Can you work these out from the model? Positions are in its coordinate system, mm. Face numbers are marked on the shaded views. A direction names the side the tool comes from. Coordinates: 2 decimals unless noted, no trailing zeros. Order: outer loops, then holes, each group sorted by start corner. A loop starts at its lowest first (then second) coordinate and runs counter-clockwise, first axis right, second up. Notation, with made-up numbers: (83, 47.5) -> (114, 47.5) arc R20 ccw to (114, 58.5) -> close; hole circle Ø4 at (-30.5, 64). An arc over 180 degrees is marked (long way). Return JSON: item names as keys, results as strings. Group by question number.
1) If I drill on probe 1 along X at (y, z) = (5, 1.6); probe 2 along Y at (x, z) = (17, 3); probe 3 along Y at (x, z) = (89, 1.1), over which ranges is the centre line in solid material (lowest first)? Write a range as from..to.
2) If we section it at A-A, the plane x = 17: Please give me the cut outline in (y, z).
3) For the marked faces 1, 2, 3 and 4, which set-ups out of +Z, -Z, +X, -X, +Y, -Y let a thin tool reach every point of the face, with its end or its side?
4) If we section it at B-B, the plane z = 3: State how many separate pieces and enclosed holes the cut face has, then the cut area to 3 significant figures.
5) For pin 1 (1.8 mm diameter, centred on x = 64, y = 58.5, fed in from +Z); pin 2 (5.5 mm diameter, centred on x = 65, y = 5, fed in from -Z); pin 3 (2.5 mm diameter, centred on x = 113, y = 60, fed in from +Z), each with a flat end and sliding along its axis, tell me the tip position at first contact or that it passes through.
6) If we section it at D-D, the plane x = 33: Please give me the cut outline in (y, z).
from build123d import *

# Parameters (mm, degrees)
ESQUISSE1_W             = 130
ESQUISSE1_H             = 65
ESQUISSE1_R             = 1.6
BOSS_EXTRU_1_DEPTH      = 5
ESQUISSE2_W             = 130
ESQUISSE2_H             = 13.5
ESQUISSE2_H_2           = 22
ENL_V_MAT_EXTRU_1_DEPTH = 0.5
ESQUISSE3_R             = 3
ENL_V_MAT_EXTRU_2_DEPTH = 3


with BuildPart() as part:
    # Esquisse1 → Boss.-Extru.1 (new body)
    with BuildSketch(Plane.XY):
        with Locations((65, 32.5)):
            Rectangle(ESQUISSE1_W, ESQUISSE1_H)
        with Locations((113, 5)):
            Circle(ESQUISSE1_R, mode=Mode.SUBTRACT)
        with Locations((89, 5)):
            Circle(ESQUISSE1_R, mode=Mode.SUBTRACT)
        with Locations((65, 5)):
            Circle(ESQUISSE1_R, mode=Mode.SUBTRACT)
        with Locations((41, 5)):
            Circle(ESQUISSE1_R, mode=Mode.SUBTRACT)
        with Locations((17, 5)):
            Circle(ESQUISSE1_R, mode=Mode.SUBTRACT)
        with Locations((113, 60)):
            Circle(ESQUISSE1_R, mode=Mode.SUBTRACT)
        with Locations((89, 60)):
            Circle(ESQUISSE1_R, mode=Mode.SUBTRACT)
        with Locations((65, 60)):
            Circle(ESQUISSE1_R, mode=Mode.SUBTRACT)
        with Locations((41, 60)):
            Circle(ESQUISSE1_R, mode=Mode.SUBTRACT)
        with Locations((17, 60)):
            Circle(ESQUISSE1_R, mode=Mode.SUBTRACT)
    extrude(amount=BOSS_EXTRU_1_DEPTH)

    # Esquisse2 → Enlèv. mat.-Extru.1 (cut)
    with BuildSketch(Plane(origin=(0, 0, 0), x_dir=(-1, 0, 0), z_dir=(0, 0, -1))):
        with Locations((-65, 58.25)):
            Rectangle(ESQUISSE2_W, ESQUISSE2_H)
        with Locations((-65, 6.75)):
            Rectangle(ESQUISSE2_W, ESQUISSE2_H)
        with Locations((-65, 32.5)):
            Rectangle(ESQUISSE2_W, ESQUISSE2_H_2)
    extrude(amount=-ENL_V_MAT_EXTRU_1_DEPTH, mode=Mode.SUBTRACT)

    # Esquisse3 → Enlèv. mat.-Extru.2 (cut)
    with BuildSketch(Plane.XY.offset(5)):
        with Locations((17, 60)):
            Circle(ESQUISSE3_R)
        with Locations((41, 60)):
            Circle(ESQUISSE3_R)
        with Locations((65, 60)):
            Circle(ESQUISSE3_R)
        with Locations((89, 60)):
            Circle(ESQUISSE3_R)
        with Locations((113, 60)):
            Circle(ESQUISSE3_R)
        with Locations((113, 5)):
            Circle(ESQUISSE3_R)
        with Locations((89, 5)):
            Circle(ESQUISSE3_R)
        with Locations((65, 5)):
            Circle(ESQUISSE3_R)
        with Locations((41, 5)):
            Circle(ESQUISSE3_R)
        with Locations((17, 5)):
            Circle(ESQUISSE3_R)
    extrude(amount=-ENL_V_MAT_EXTRU_2_DEPTH, mode=Mode.SUBTRACT)


solid = part.part
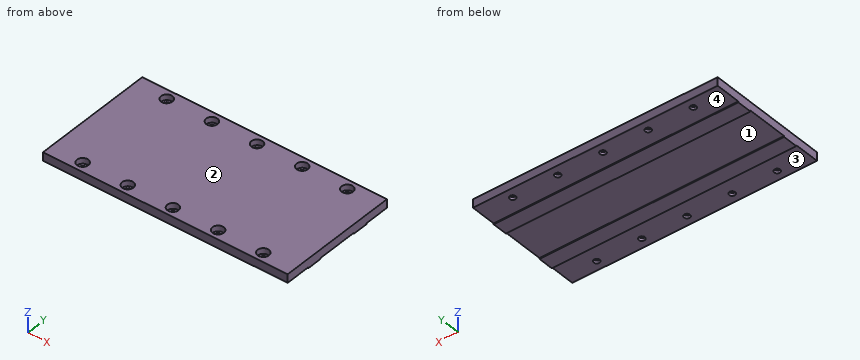
Result sheet:
{
 "1": {"probe 1": "x = 0..15.4, 18.6..39.4, 42.6..63.4, 66.6..87.4, 90.6..111.4, 114.6..130", "probe 2": "y = 0..2, 8..57, 63..65", "probe 3": "y = 0..3.4, 6.6..58.4, 61.6..65"},
 "2": {"outline": "(0, 0.5) -> (3.4, 0.5) -> (3.4, 2) -> (2, 2) -> (2, 5) -> (0, 5) -> close; (6.6, 0.5) -> (13.5, 0.5) -> (13.5, 0) -> (21.5, 0) -> (21.5, 0.5) -> (43.5, 0.5) -> (43.5, 0) -> (51.5, 0) -> (51.5, 0.5) -> (58.4, 0.5) -> (58.4, 2) -> (57, 2) -> (57, 5) -> (8, 5) -> (8, 2) -> (6.6, 2) -> close; (61.6, 0.5) -> (65, 0.5) -> (65, 5) -> (63, 5) -> (63, 2) -> (61.6, 2) -> close"},
 "3": {"face 1": "-Z, +X, -X", "face 2": "+Z, +X, -X, +Y, -Y", "face 3": "-Z, +X, -X, -Y", "face 4": "-Z, +X, -X, +Y"},
 "4": {"separate pieces": "1", "enclosed holes": "10", "area": "8,170 mm2"},
 "5": {"pin 1": "stops at z = 2", "pin 2": "stops at z = 0.5", "pin 3": "passes through"},
 "6": {"outline": "(0, 0.5) -> (13.5, 0.5) -> (13.5, 0) -> (21.5, 0) -> (21.5, 0.5) -> (43.5, 0.5) -> (43.5, 0) -> (51.5, 0) -> (51.5, 0.5) -> (65, 0.5) -> (65, 5) -> (0, 5) -> close"}
}
